The listing builds one solid part. Answer for the finished solid, in the listing's coordinates (mm). Face numbers are marked on the shaded views. Coordinates: 2 decimals unless noted, no trailing zeros. Order: outer loops, then holes, each group sorted by start corner. A loop starts at its lowest first (then second) coordinate and runs counter-clockwise, first axis right, second up. Notation, with made-up numbers: (50.25, 47) -> (92.25, 47) arc R23 ccw to (92.25, 61) -> close; hole circle Ø8 at (-14.75, -30). An arc over 180 degrees is marked (long way). Return JSON: item names as keys, results as strings.
from build123d import *

# Parameters (mm, degrees)
F1_DEPTH = 1500
F3_DEPTH = 76.201


with BuildPart() as f1:
    # F0 (on Front) → F1 (new body)
    with BuildSketch(Plane.XZ):
        with BuildLine():
            Line((73, 108.31944), (0, 108.31944))
            Line((0, 108.31944), (-73, 108.31944))
            Line((-73, 108.31944), (-73, 97.41944))
            Line((-73, 97.41944), (-13.2, 97.41944))
            ThreePointArc((-13.2, 97.41944), (-6.128932, 94.490508), (-3.2, 87.41944))
            Line((-3.2, 87.41944), (-3.2, -126.78056))
            ThreePointArc((-3.2, -126.78056), (-6.128932, -133.851628), (-13.2, -136.78056))
            Line((-13.2, -136.78056), (-73, -136.78056))
            Line((-73, -136.78056), (-73, -147.68056))
            Line((-73, -147.68056), (0, -147.68056))
            Line((0, -147.68056), (73, -147.68056))
            Line((73, -147.68056), (73, -136.78056))
            Line((73, -136.78056), (13.2, -136.78056))
            ThreePointArc((13.2, -136.78056), (6.128932, -133.851628), (3.2, -126.78056))
            Line((3.2, -126.78056), (3.2, 87.41944))
            ThreePointArc((3.2, 87.41944), (6.128932, 94.490508), (13.2, 97.41944))
            Line((13.2, 97.41944), (73, 97.41944))
            Line((73, 97.41944), (73, 108.31944))
        make_face()
    extrude(amount=-F1_DEPTH)

    # F2 (on face) → F3 (cut, through all)
    with BuildSketch(Plane.YZ.offset(3.2)):
        with BuildLine():
            Line((475, 37.5), (210, 37.5))
            ThreePointArc((210, 37.5), (202.928932, 34.571068), (200, 27.5))
            Line((200, 27.5), (200, -27.5))
            ThreePointArc((200, -27.5), (202.928932, -34.571068), (210, -37.5))
            Line((210, -37.5), (475, -37.5))
            ThreePointArc((475, -37.5), (482.071068, -34.571068), (485, -27.5))
            Line((485, -27.5), (485, 27.5))
            ThreePointArc((485, 27.5), (482.071068, 34.571068), (475, 37.5))
        make_face()
        with BuildLine():
            Line((1290, 37.5), (1025, 37.5))
            ThreePointArc((1025, 37.5), (1017.928932, 34.571068), (1015, 27.5))
            Line((1015, 27.5), (1015, -27.5))
            ThreePointArc((1015, -27.5), (1017.928932, -34.571068), (1025, -37.5))
            Line((1025, -37.5), (1290, -37.5))
            ThreePointArc((1290, -37.5), (1297.071068, -34.571068), (1300, -27.5))
            Line((1300, -27.5), (1300, 27.5))
            ThreePointArc((1300, 27.5), (1297.071068, 34.571068), (1290, 37.5))
        make_face()
    extrude(amount=-F3_DEPTH, mode=Mode.SUBTRACT)


solid = f1.part
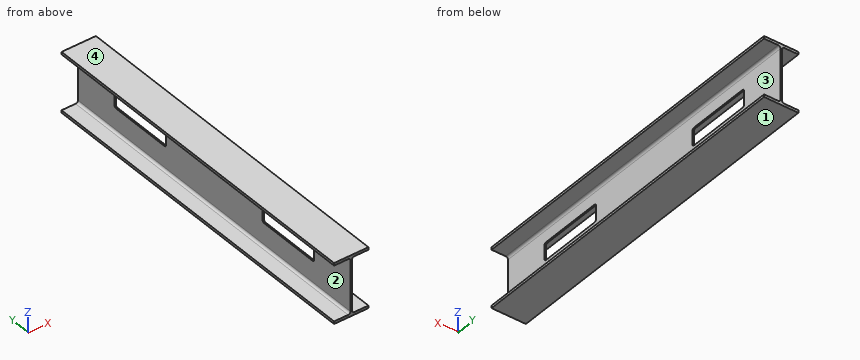
1. Determine the mould class of the marked faces 1, 2, 3 and 4 for opening direction Z: pulls with the +Z half, pulls with the -Z half, needs draft (parallel to the pull), parting line crosses it, or undercut.
Answer block:
{"face 1": "pulls with the -Z half", "face 2": "undercut", "face 3": "undercut", "face 4": "pulls with the +Z half"}
2. The part is cut by section C-C on y = 565.5. Give the vertices of the cut face in (x, z), and give its area (3 significant figures).
Answer block:
{"outline": "(-73, -147.68) -> (73, -147.68) -> (73, -136.78) -> (13.2, -136.78) arc R10 cw to (3.2, -126.78) -> (3.2, 87.42) arc R10 cw to (13.2, 97.42) -> (73, 97.42) -> (73, 108.32) -> (-73, 108.32) -> (-73, 97.42) -> (-13.2, 97.42) arc R10 cw to (-3.2, 87.42) -> (-3.2, -126.78) arc R10 cw to (-13.2, -136.78) -> (-73, -136.78) -> close", "area": "4,770 mm2"}
3. The part is cut by section A-A on x = 36. Give the vertices of the cut face in (y, z), and give its area (3 significant figures).
Answer block:
{"outline": "(0, -147.68) -> (1500, -147.68) -> (1500, -136.78) -> (0, -136.78) -> close; (0, 97.42) -> (1500, 97.42) -> (1500, 108.32) -> (0, 108.32) -> close", "area": "32,700 mm2"}
4. The part is cut by section D-D on z = -81. Give the vertices of the cut face in (x, y), and give its area (3 significant figures).
Answer block:
{"outline": "(-3.2, 0) -> (3.2, 0) -> (3.2, 1500) -> (-3.2, 1500) -> close", "area": "9,600 mm2"}
5. This flat-tipped pin is pushed along its axis until it touches: pin 1 Ø1.5 at (y, z) = (747.5, -68) entering from +X. Where does it stop, or does it pass through?
Answer block:
{"pin 1": "stops at x = 3.2"}
6. The part is cut by section B-B on y = 1270. Give the vertices of the cut face in (x, z), and give its area (3 significant figures).
Answer block:
{"outline": "(-73, -147.68) -> (73, -147.68) -> (73, -136.78) -> (13.2, -136.78) arc R10 cw to (3.2, -126.78) -> (3.2, -37.5) -> (-3.2, -37.5) -> (-3.2, -126.78) arc R10 cw to (-13.2, -136.78) -> (-73, -136.78) -> close; (-73, 97.42) -> (-13.2, 97.42) arc R10 cw to (-3.2, 87.42) -> (-3.2, 37.5) -> (3.2, 37.5) -> (3.2, 87.42) arc R10 cw to (13.2, 97.42) -> (73, 97.42) -> (73, 108.32) -> (-73, 108.32) -> close", "area": "4,290 mm2"}
7. Consider line 1 (Z direction, x = -25.5, y = 301); line 2 (X direction, y = 789, z = 71); line 3 (Z direction, x = -1, y = 321.5). Determine where each line is inside the solid, lowest interval first. Write a range as from..to.
Answer block:
{"line 1": "z = -147.68..-136.78, 97.42..108.32", "line 2": "x = -3.2..3.2", "line 3": "z = -147.68..-37.5, 37.5..108.32"}
